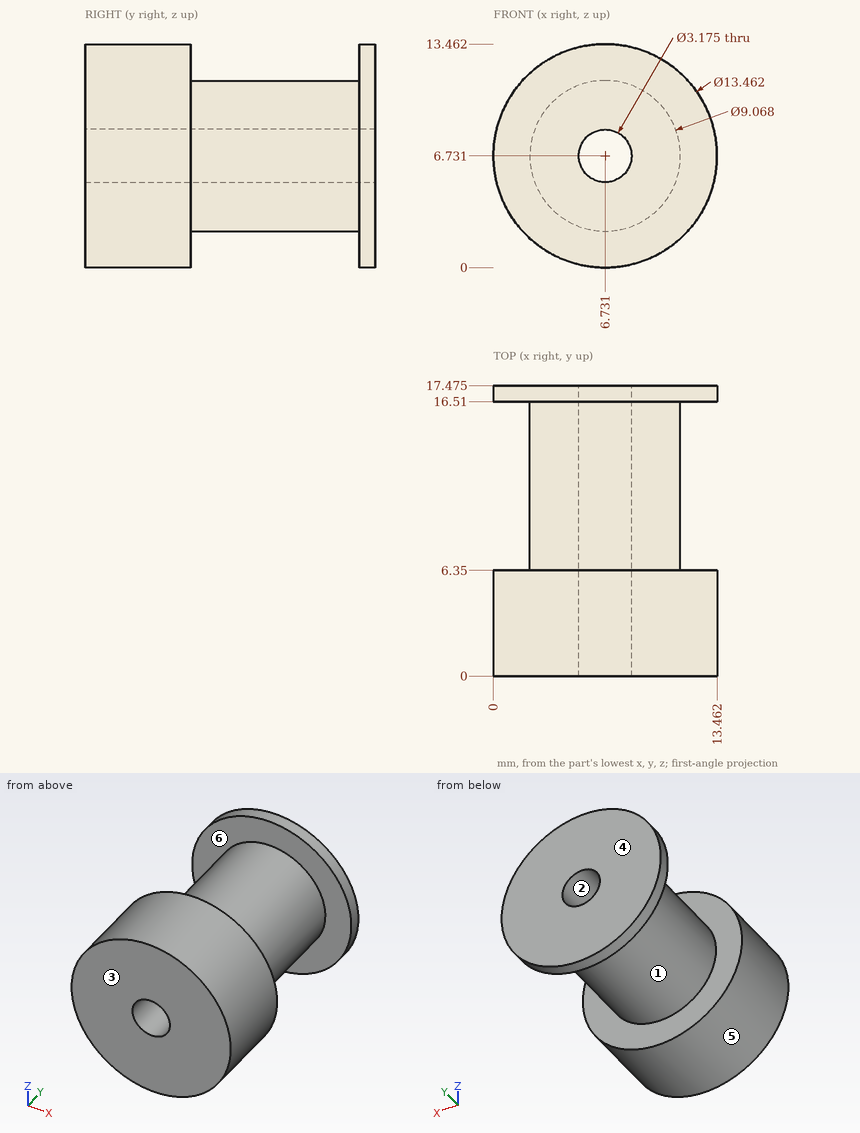
Can you work these out from the drawing? Everything is in mm from the part's minimum corner. A direction names the side the tool comes from. Coordinates: 2 decimals unless noted, no trailing zeros. One line per item, written item: value.
1. Will these pins go through, and if not, where does the flat tip stop? pin 1 Ø4 at (x, y) = (11, 5) entering from -Z; pin 2 Ø5 at (x, y) = (3, 4) entering from +Z; pin 3 Ø4 at (y, z) = (10.5, 3) entering from -X.
Geometry says:
pin 1: stops at z = 0.39
pin 2: stops at z = 13.35
pin 3: stops at x = 2.54
2. Please list where these lines run through material, in increasing order: probe 1 along Z at (x, y) = (6, 13.5) (1 decimal); probe 2 along X at (y, z) = (8, 7.25) (1 decimal); probe 3 along X at (y, z) = (1, 7.75) (1 decimal).
Geometry says:
probe 1: z = 2.3 to 5.3, 8.1 to 11.2
probe 2: x = 2.2 to 5.2, 8.2 to 11.2
probe 3: x = 0.1 to 5.5, 7.9 to 13.4
3. Thinking about a two-plate mould opening in Y: for the marked faces 1, 2, 3 and 4, which applies, +Y half, -Y half, draft (parallel to the pull), parting line (faces both ways), or undercut?
Geometry says:
face 1: undercut
face 2: draft
face 3: -Y half
face 4: +Y half
4. On a 3-axis mill with a long thin cutter (end or side, diameter ignored), from which of +Z, -Z, +X, -X, +Y, -Y can I reach the whole of each face in a straight line? I mean the marked faces 5 and 6. Say none if no direction works.
Geometry says:
face 5: +Y, -Y
face 6: none
